Geometry check sheet. Reference: the model listing, model coordinates, mm. A direction names the side the tool comes from. Give positions to 0.01 mm unless a question says otherwise; leave off trailing zeros. Loops run counter-clockwise (first coordinate to the right, second up) from the corner with the lowest first, then second, coordinate; pieces in that order, holes last.
Autodesk Inventor part; units mm, degrees
ref_plane "YZ Plane" through (0, 0, 0) normal (1, 0, 0) x (0, 1, 0)
ref_plane "XZ Plane" through (0, 0, 0) normal (0, 1, 0) x (-1, 0, 0)
ref_plane "XY Plane" through (0, 0, 0) normal (0, 0, 1) x (1, 0, 0)
sketch "Эскиз1" plane through (0, 0, 0) normal (0, 0, 1) x (1, 0, 0)
  line L0 (10.0582, -8.8009) -> (-16.8718, -8.8009)
  line L1 (-16.8718, -8.8009) -> (-16.8718, 8.0709)
  line L2 (-16.8718, 8.0709) -> (10.0582, 8.0709)
  line L3 (10.0582, 8.0709) -> (10.0582, -8.8009)
  point P0 (0, 0)
extrude "Выдавливание1" add sketch "Эскиз1" along normal blind 10
sketch "Эскиз2" plane through (0, 0, 10) normal (0, 0, 1) x (1, 0, 0)
  circle A0 centre (4.6641, -5.9619) radius 1
  circle A1 centre (-14.4383, -5.9619) radius 1
  point P0 (0, 0)
  dimension "d2" = 2
  dimension "d3" = 2
extrude "Выдавливание2" add sketch "Эскиз2" along normal blind 2
sketch "Эскиз3" plane through (4.6641, -5.9619, 12) normal (0, 0, 1) x (1, 0, 0)
  circle A0 centre (0, 0) radius 1
  circle A1 centre (0, 0) radius 2
  circle A2 centre (-14.7836, -12.664) radius 2
  line L0 (-1.2061, 1.5954) -> (-15.8126, -10.949)
  line L1 (-13.5836, -14.264) -> (1.0265, -1.7165)
  point P0 (-4.6641, 5.9619)
  dimension "d6" = 4
  dimension "d7" = 4
extrude "Выдавливание3" add sketch "Эскиз3" along normal blind 2
sketch "Эскиз4" plane through (-14.4383, -5.9619, 12) normal (0, 0, 1) x (1, 0, 0)
  circle A0 centre (0, 0) radius 1
  point P0 (14.4383, 5.9619)
extrude "Выдавливание4" add sketch "Эскиз4" along normal blind 4
sketch "Эскиз5" plane through (4.6641, -5.9619, 14) normal (0, 0, 1) x (1, 0, 0)
  circle A0 centre (-10.7969, -8.6603) radius 1
  point P0 (-4.6641, 5.9619)
  dimension "d12" = 2
extrude "Выдавливание5" add sketch "Эскиз5" along normal blind 2
sketch "Эскиз6" plane through (4.6641, -5.9619, 14) normal (0, 0, 1) x (1, 0, 0)
  circle A0 centre (-15.0265, -12.7992) radius 1
  point P0 (-4.6641, 5.9619)
  dimension "d15" = 2
extrude "Выдавливание6" cut sketch "Эскиз6" against normal blind 10
sketch "Эскиз7" plane through (-14.4383, -5.9619, 16) normal (0, 0, 1) x (1, 0, 0)
  circle A0 centre (0, 0) radius 2
  circle A1 centre (8.3055, -8.6603) radius 1
  circle A2 centre (8.3055, -8.6603) radius 2
  line L0 (7.3055, -6.9282) -> (1.7093, -1.0384)
  line L1 (6.6268, -7.5731) -> (1.0492, -1.7027)
  point P0 (14.4383, 5.9619)
  dimension "d18" = 4
  dimension "d19" = 4
extrude "Выдавливание7" add sketch "Эскиз7" along normal blind 2 contours A0 | A0 L0 A2 L1 | A2 | A1
sketch "Эскиз8" plane through (-14.4383, -5.9619, 18) normal (0, 0, 1) x (1, 0, 0)
  circle A0 centre (0, 0) radius 1
  point P0 (14.4383, 5.9619)
extrude "Выдавливание8" cut sketch "Эскиз8" against normal blind 1
chamfer "Фаска1" distance 0.3 angle 45 4 edges at (-9.9309, -9.9452, 18) (-9.9309, -9.9452, 16) (-10.6004, -10.5998, 16) (-10.6004, -10.5998, 18)
1) Depth check by flat-ended pin: P1, Ø8.5, axis at x = -1, y = -15.5, coming from the -Z side; P2, Ø4, axis at x = -4.5, y = -8.5, coming from the +Z side; P3, Ø5, axis at x = -8.5, z = 5, coming from the -Y side. Enter the tip coordinate at first touch or a pass-through.
2) Sectioned sample at A-A on x = 2.75. Enter the section's corners in (y, z), plus the area to 3 significant figures.
3) Sectioned sample at C-C on z = 10.5. Enter the section's corners in (x, y), plus the area to 3 significant figures.
4) Sectioned sample at D-D on x = -14. Enter the section's corners in (y, z).
5) Mould release check, pull along Z, two halves, no side actions. Record for faces 1 (the flat face through (-3, -8.801, 5)), 2 (the cylindrical face through (4.534, -6.953, 10.986)), 3 (the flat face through (-14, -6, 17)), 4 (the flat face through (-3, -12, 12)): +Z half, -Z half, draft (parallel to the pull), parting line (faces both ways), or undercut.
6) Sectioned sample at B-B on y = -12.25. Enter the section's corners in (x, z), plus the area to 3 significant figures.
7) Tool access check on faces 5 (the flat face through (-16.872, 0, 5)), 6 (the cylindrical face through (-14.568, -6.953, 12.958)), 7 (the cylindrical face through (6.3, -4.81, 12.99)). Record the directions out of +Z, -Z, +X, -X, +Y, -Y that give a thin tool (end or side, any length) a straight path to the whole face; none if there is none.
8) Scan lines: line 1 along Z through (x, y) = (-6.25, 2.75); line 2 along Y through (x, z) = (-3.75, 4); line 3 along Z through (x, y) = (0, -11). Record each from-to range of solid material in increasing order.
Determined:
1. P1: stops at z = 12
1. P2: stops at z = 10
1. P3: stops at y = -8.8
2. outline: (-10.2, 12) - (-4.97, 12) - (-4.97, 14) - (-10.2, 14) - close; (-8.8, 0) - (8.07, 0) - (8.07, 10) - (-8.8, 10) - close
2. area: 179 mm2
3. outline: circle Ø2 at (-14.44, -5.96); circle Ø2 at (4.66, -5.96)
3. area: 6.28 mm2
4. outline: (-8.8, 0) - (8.07, 0) - (8.07, 10) - (-5.06, 10) - (-5.06, 16) - (-4.01, 16) - (-4.01, 18) - (-5.06, 18) - (-5.06, 17) - (-6.86, 17) - (-6.86, 18) - (-7.91, 18) - (-7.91, 16) - (-6.86, 16) - (-6.86, 10) - (-8.8, 10) - close
5. face 1: draft
5. face 2: undercut
5. face 3: +Z half
5. face 4: undercut
6. outline: (-9.03, 16.3) - (-8.62, 16) - (-8.15, 16) - (-7.74, 16.3) - (-7.74, 17.7) - (-8.15, 18) - (-8.62, 18) - (-9.03, 17.7) - close; (-5.72, 12) - (0.37, 12) - (0.37, 14) - (-5.72, 14) - close
6. area: 14.5 mm2
7. face 5: +Z, -Z, -X, +Y, -Y
7. face 6: none
7. face 7: +Z
8. line 1: z = 0 to 10
8. line 2: y = -8.8 to 8.07
8. line 3: z = 12 to 14
